Source: three-view drawing plus pictorial views. Frame: mm from the lowest corner of the part. A direction names the side the tool comes from. Coordinates: 2 decimals unless noted, no trailing zeros. Order: outer loops, then holes, each group sorted by start corner. A loop starts at its lowest first (then second) coordinate and runs counter-clockwise, first axis right, second up. Notation, with made-up numbers: M 84.25,24.25 L 135.25,24.25 A20 cw 135.25,33.25 Z; hole C 49,35.5 d4. An arc over 180 degrees is marked long. Use CSV: the item, a comma, the result in double quotes. Start each with the question number.
Q1. Section query C-C, the plane z = 5.5. Output: boundary loops of the cut face in (x, y), and give its area (3 significant figures).
Q2. Ray query, probe 1 along Z at (x, y) = (35.5, 15); probe 2 along X at (y, z) = (8, 5); probe 3 along Y at (x, z) = (15, 7.25). Return the intervals inside material, ascending.
Q3. First-contact query: P1, Ø12, axis at x = 27, z = 9, coming from the -Y side; P2, Ø3, axis at x = 17.5, z = 16.5, coming from the +Y side. Flat tips, straight axial feed; report the tip coordinate or a pass-through.
Q4. Section query A-A, the plane y = 15. Output: boundary loops of the cut face in (x, z).
Q5. Mould query, pull axis X, two halves, no side actions, for the marked faces 1, 2, 3 and 4. Classes: +X half, -X half, draft (parallel to the pull), parting line (faces both ways), or undercut.
Q6. Section query D-D, the plane y = 18.75. Output: boundary loops of the cut face in (x, z).
Q7. Section query B-B, the plane z = 13. Output: boundary loops of the cut face in (x, y).
Q8. Access query for the marked faces 5 and 6. Directions: +Z, -Z, +X, -X, +Y, -Y. A direction counts if a zero-diameter tool reaches every point of the face in a straight line with its end or side. Return the directions, or none.
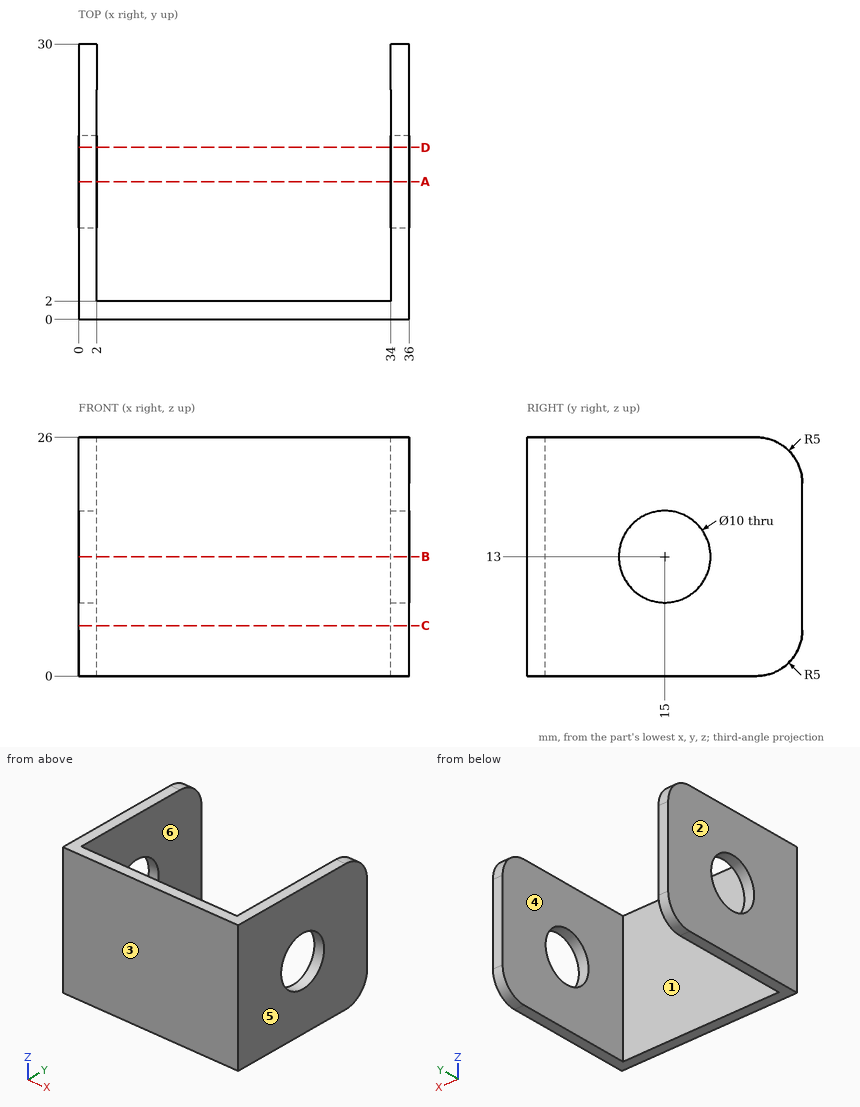
Responses:
1,outline,"M 0,0 L 36,0 L 36,30 L 34,30 L 34,2 L 2,2 L 2,30 L 0,30 Z"
1,area,"184 mm²"
2,probe 1,"z = 0 to 8, 18 to 26"
2,probe 2,"x = 0 to 2, 34 to 36"
2,probe 3,"y = 0 to 2"
3,P1,"stops at y = 0"
3,P2,"stops at y = 2"
4,outline,"M 0,0 L 2,0 L 2,8 L 0,8 Z; M 0,18 L 2,18 L 2,26 L 0,26 Z; M 34,0 L 36,0 L 36,8 L 34,8 Z; M 34,18 L 36,18 L 36,26 L 34,26 Z"
5,face 1,"undercut"
5,face 2,"-X half"
5,face 3,"draft"
5,face 4,"undercut"
6,outline,"M 0,0 L 2,0 L 2,9.69 L 0,9.69 Z; M 0,16.31 L 2,16.31 L 2,26 L 0,26 Z; M 34,0 L 36,0 L 36,9.69 L 34,9.69 Z; M 34,16.31 L 36,16.31 L 36,26 L 34,26 Z"
7,outline,"M 0,0 L 36,0 L 36,10 L 34,10 L 34,2 L 2,2 L 2,10 L 0,10 Z; M 0,20 L 2,20 L 2,30 L 0,30 Z; M 34,20 L 36,20 L 36,30 L 34,30 Z"
8,face 5,"+Z, -Z, +X, +Y, -Y"
8,face 6,"+Z, -Z, +Y"
